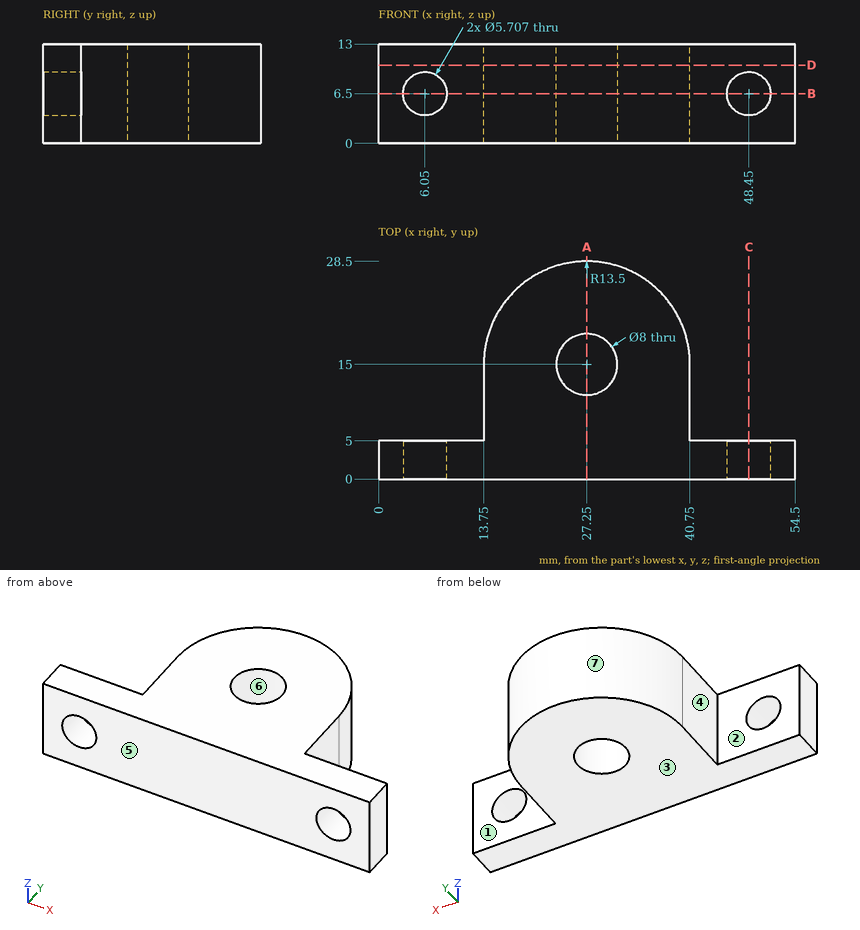
Check sheet for the drawn part. Datum: minimum x, y, z corner. Units: mm. A direction names the side the tool comes from. Give positions to 0.01 mm unless a question says otherwise; leave off trailing zeros. Write each loop counter-clockwise with the first axis right and the second up, starting at its lowest first coordinate (ties: lowest second). Pieces come first, ordered by that corner, then holes. Notation, with made-up numbers: (-9.75, 64.5) - (37.25, 64.5) arc R34 ccw to (37.25, 97.5) - close; hole circle Ø5 at (48, 12). An arc over 180 degrees is marked (long way). Put each result on its own line as item: value.
1. Sectioned sample at B-B, the plane z = 6.5. Enter the section's corners in (x, y).
Ans:
outline: (0, 0) - (3.2, 0) - (3.2, 5) - (0, 5) - close; (8.9, 0) - (45.6, 0) - (45.6, 5) - (40.75, 5) - (40.75, 15) arc R13.5 ccw to (13.75, 15) - (13.75, 5) - (8.9, 5) - close; (51.3, 0) - (54.5, 0) - (54.5, 5) - (51.3, 5) - close; hole circle Ø8 at (27.25, 15)
2. Sectioned sample at C-C, the plane x = 48.45. Enter the section's corners in (y, z).
Ans:
outline: (0, 0) - (5, 0) - (5, 3.65) - (0, 3.65) - close; (0, 9.35) - (5, 9.35) - (5, 13) - (0, 13) - close
3. Set-up check for the marked faces 1, 2 and 3: record each of +Z, -Z, +X, -X, +Y, -Y from which the full face is reachable in a straight line by a thin tool's end or side.
Ans:
face 1: +Z, -Z, +X, +Y
face 2: +Z, -Z, -X, +Y
face 3: -Z, +X, -X, +Y, -Y
4. Sectioned sample at D-D, the plane z = 10.25. Enter the section's corners in (x, y).
Ans:
outline: (0, 0) - (54.5, 0) - (54.5, 5) - (40.75, 5) - (40.75, 15) arc R13.5 ccw to (13.75, 15) - (13.75, 5) - (0, 5) - close; hole circle Ø8 at (27.25, 15)
5. Draft check along Y on the marked faces 4, 5, 6 and 7. Enter one of: +Y half, -Y half, draft (parallel to the pull), parting line (faces both ways), or undercut.
Ans:
face 4: draft
face 5: -Y half
face 6: undercut
face 7: +Y half
6. Go/stop test with flat-tipped pins: pin 1 (5 mm diameter, centred on x = 11, z = 10.5, fed in from +Y); pin 2 (1.5 mm diameter, centred on x = 12.5, y = 18, fed in from -Z); pin 3 (1.5 mm diameter, centred on y = 9, z = 3, fed in from +X); pin 4 (3 mm diameter, centred on y = 7.5, z = 10, fed in from -X). Record where each tip stops, or that it passes through.
Ans:
pin 1: stops at y = 5
pin 2: passes through
pin 3: stops at x = 40.75
pin 4: stops at x = 13.75
7. Thickness scan on line 1 (X direction, y = 15, z = 3.75); line 2 (Z direction, x = 48.45, y = 1.3); line 3 (Z direction, x = 48, y = 4). Record the ranges inside material, lowest first.
Ans:
line 1: x = 13.75 to 23.25, 31.25 to 40.75
line 2: z = 0 to 3.65, 9.35 to 13
line 3: z = 0 to 3.68, 9.32 to 13
8. Sectioned sample at A-A, the plane x = 27.25. Enter the section's corners in (y, z).
Ans:
outline: (0, 0) - (11, 0) - (11, 13) - (0, 13) - close; (19, 0) - (28.5, 0) - (28.5, 13) - (19, 13) - close
